```python
from build123d import *

# Parameters (mm, degrees)
SKETCH1_W                                    = 60
SKETCH1_H                                    = 60
BOSS_EXTRUDE1_DEPTH                          = 14.5
CBORE_FOR_M8_HEX_SOCKET_HEAD_CAP_SCR_2_COUNT = 2
CBORE_FOR_M8_HEX_SOCKET_HEAD_CAP_SCR_2_PITCH = 30
CBORE_FOR_M8_HEX_SOCKET_HEAD_CAP_SCR_3_COUNT = 2
CBORE_FOR_M8_HEX_SOCKET_HEAD_CAP_SCR_3_PITCH = 42.426406871
CBORE_FOR_M8_HEX_SOCKET_HEAD_CAP_SCR_4_COUNT = 2
CBORE_FOR_M8_HEX_SOCKET_HEAD_CAP_SCR_4_PITCH = 30
FILLET1_R                                    = 2
CHAMFER1_SIZE                                = 0.5


with BuildPart() as part:
    # Sketch1 → Boss-Extrude1 (new body)
    with BuildSketch(Plane(origin=(0, 0, 0), x_dir=(1, 0, 0), z_dir=(0, 1, 0))):
        Rectangle(SKETCH1_W, SKETCH1_H)
    extrude(amount=BOSS_EXTRUDE1_DEPTH)

    # Sketch4 → CBORE for M8 Hex Socket Head Cap Screw1 (revolve, cut)
    with BuildSketch(Plane(origin=(-15, 14.5, 15), x_dir=(0, 0, 1), z_dir=(1, 0, 0))):
        Polygon((0, 0), (0, 14.5), (5, 14.5), (4.5, 14), (4.5, 8.6), (7.5, 8.6), (7.5, 0.5), (8, 0), align=None)
    cbore_for_m8_hex_socket_head_cap_screw1 = revolve(axis=Axis((-15, 20.85, 15), (0, -1, 0)), mode=Mode.SUBTRACT)

    # CBORE for M8 Hex Socket Head Cap Scr 2: CBORE for M8 Hex Socket Head Cap Screw1 ×2
    with Locations(*[(i * CBORE_FOR_M8_HEX_SOCKET_HEAD_CAP_SCR_2_PITCH, 0, 0) for i in range(1, CBORE_FOR_M8_HEX_SOCKET_HEAD_CAP_SCR_2_COUNT)]):
        add(cbore_for_m8_hex_socket_head_cap_screw1, mode=Mode.SUBTRACT)

    # CBORE for M8 Hex Socket Head Cap Scr 3: CBORE for M8 Hex Socket Head Cap Screw1 ×2
    with Locations(*[Vector(0.7071067811865476, 0, -0.7071067811865476) * (i * CBORE_FOR_M8_HEX_SOCKET_HEAD_CAP_SCR_3_PITCH) for i in range(1, CBORE_FOR_M8_HEX_SOCKET_HEAD_CAP_SCR_3_COUNT)]):
        add(cbore_for_m8_hex_socket_head_cap_screw1, mode=Mode.SUBTRACT)

    # CBORE for M8 Hex Socket Head Cap Scr 4: CBORE for M8 Hex Socket Head Cap Screw1 ×2
    with Locations(*[(0, 0, -i * CBORE_FOR_M8_HEX_SOCKET_HEAD_CAP_SCR_4_PITCH) for i in range(1, CBORE_FOR_M8_HEX_SOCKET_HEAD_CAP_SCR_4_COUNT)]):
        add(cbore_for_m8_hex_socket_head_cap_screw1, mode=Mode.SUBTRACT)

    # Sketch7 → M12 Tapped Hole1 (revolve, cut)
    with BuildSketch(Plane(origin=(0, 14.5, 0), x_dir=(0, 0, 1), z_dir=(1, 0, 0))):
        Polygon((0, 0), (0, 14.5), (6, 14.5), (5.1, 13.6), (5.1, 0.9), (6, 0), align=None)
    revolve(axis=Axis((0, 20.85, 0), (0, -1, 0)), mode=Mode.SUBTRACT)

    # Fillet1
    fillet1_edges = [part.edges().sort_by_distance(p)[0] for p in [
        (-30, 7.25, -30),
        (30, 7.25, -30),
        (30, 7.25, 30),
        (-30, 7.25, 30),
    ]]
    fillet(fillet1_edges, radius=FILLET1_R)

    # Chamfer1
    chamfer1_edges = [part.edges().sort_by_distance(p)[0] for p in [
        (0, 0, 30),
        (0, 14.5, 30),
        (-30, 0, 0),
        (0, 0, -30),
        (30, 0, 0),
        (-29.414213562, 0, -29.414213562),
        (29.414213562, 0, -29.414213562),
        (29.414213562, 0, 29.414213562),
        (-29.414213562, 0, 29.414213562),
        (-30, 14.5, 0),
        (30, 14.5, 0),
        (0, 14.5, -30),
        (-29.414213562, 14.5, -29.414213562),
        (29.414213562, 14.5, -29.414213562),
        (29.414213562, 14.5, 29.414213562),
        (-29.414213562, 14.5, 29.414213562),
    ]]
    chamfer(chamfer1_edges, length=CHAMFER1_SIZE)


solid = part.part
```
Design review of the part built by this model. Coordinates are the model's own, in mm. A direction names the side the tool comes from. Coordinates: 2 decimals unless noted, no trailing zeros. Order: outer loops, then holes, each group sorted by start corner. A loop starts at its lowest first (then second) coordinate and runs counter-clockwise, first axis right, second up. Notation, with made-up numbers: M 28,-21 L 68,-21 A32 ccw 68,11 Z; hole C 80.5,61 d3. An arc over 180 degrees is marked long. Answer as a JSON object with one key per item and string values. Group by question number.
1) Add section A-A, the plane z = 0. Write out the cut boundary in (x, y), then the cut area to 3 significant figures.
2) For pin 1 (8 mm diameter, centred on x = 15, z = 15, fed in from +Y); pin 2 (7.5 mm diameter, centred on x = -16.5, z = 16, fed in from +Y), all flat-tipped, find the tip position at first contact; note any pin that passes through.
3) Wall thickness on L1, parallel to X at y = 4.65, z = -15; L2, parallel to X at y = 11.25, z = -14.5: over which ranges is each line inside the solid? List them lowest first.
4) Tool access review of faces 4 (the cylindrical face through (-18.04, 3.24, -18.32)), 5 (the flat face through (15, 5.9, -20)): name each direction out of +Z, -Z, +X, -X, +Y, -Y from which nothing blocks a thin tool from reaching the whole face with its end or side.
5) Add section B-B, the plane z = 15. Count the separate pieces of the cut face and the enclosed holes in it, then the cut area to 3 significant figures.
6) Mouldability with a two-part tool opening along Z and no side actions: class faces 1 (the flat face through (0, 7, 30)), 2 (the cylindrical face through (8.676, 10.007, -10.968)), 3 (the conical face through (-29.15, 0.14, -29.17)) as pulls with the +Z half, pulls with the -Z half, needs draft (parallel to the pull), parting line crosses it, or undercut.
Computed values:
{
 "1": {"outline": "M -30,0.5 L -29.5,0 L -6,0 L -5.1,0.9 L -5.1,13.6 L -6,14.5 L -29.5,14.5 L -30,14 Z; M 5.1,0.9 L 6,0 L 29.5,0 L 30,0.5 L 30,14 L 29.5,14.5 L 6,14.5 L 5.1,13.6 Z", "area": "720 mm^2"},
 "2": {"pin 1": "passes through", "pin 2": "stops at y = 5.9"},
 "3": {"L1": "x = -30 to -19.5, -10.5 to 10.5, 19.5 to 30", "L2": "x = -30 to -22.48, -7.52 to 7.52, 22.48 to 30"},
 "4": {"face 4": "+Y, -Y", "face 5": "+Y"},
 "5": {"separate pieces": "3", "enclosed holes": "0", "area": "504 mm^2"},
 "6": {"face 1": "pulls with the +Z half", "face 2": "undercut", "face 3": "pulls with the -Z half"}
}
